Source: CAD feature listing. Evaluate the final solid. Frame: model axes, mm. Face numbers are marked on the shaded views. A direction names the side the tool comes from. Give positions to 0.01 mm unless a question says otherwise; leave off trailing zeros. Order: outer loops, then holes, each group sorted by start corner. A loop starts at its lowest first (then second) coordinate and runs counter-clockwise, first axis right, second up. Notation, with made-up numbers: M 87,34 L 129,34 A15 ccw 129,47 Z; hole C 64.25,20.5 d8. An arc over 180 degrees is marked long. Use CSV: the item, a comma, the result in double quotes. Start each with the question number.
Item 1: Pull-direction query (X, two-part tool) for the marked faces 1, 2, 3 and 4; classes: +X half, -X half, draft (parallel to the pull), parting line (faces both ways), or undercut.
Item 2: Section query C-C on x = 15. Count the separate pieces of the cut face and the enclosed holes in it, and give its area (3 significant figures).
Item 3: Access query for the marked faces 5, 6 and 7. Directions: +Z, -Z, +X, -X, +Y, -Y. A direction counts if a zero-diameter tool reaches every point of the face in a straight line with its end or side. Return the directions, or none.
Item 4: Section query B-B on y = -11.5. Return loops of the section in (x, z).
Item 5: Ray query, probe 1 along X at (y, z) = (-11.5, 1.3); probe 2 along Y at (x, z) = (0, 2.3); probe 3 along Y at (x, z) = (1, 2). Return the intervals inside material, ascending. Write a range as from..to.
Item 6: Section query A-A on x = -15.5. Return loops of the section in (y, z), and give its area (3 significant figures).
Item 7: First-contact query: pin 1 (4 mm diameter, centred on x = 10.5, y = -21.5, fed in from -Z); pin 2 (4.5 mm diameter, centred on x = 15.5, y = 19.5, fed in from +Z); pin 3 (4 mm diameter, centred on x = -15.5, y = -11.5, fed in from -Z); pin 4 (3 mm diameter, centred on x = 15.5, y = -11.5, fed in from -Z). Flat tips, straight axial feed; report the tip coordinate or a pass-through.
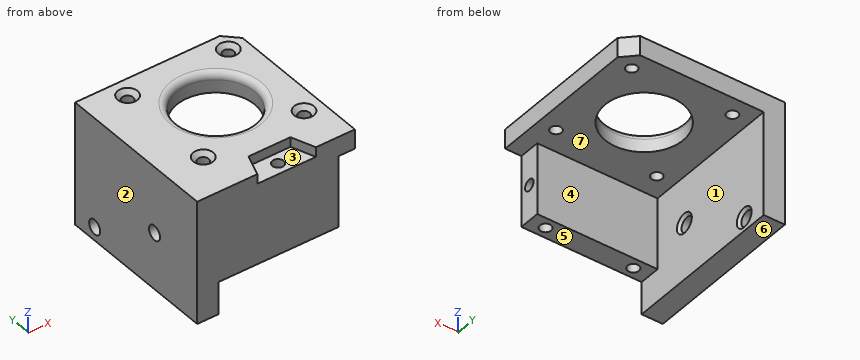
from build123d import *

# Parameters (mm, degrees)
SKETCH028_W         = 6.5
SKETCH028_H         = 50
PAD010_DEPTH        = 6
PAD010_DEPTH_BACK   = 32
HOLE011_D           = 4.5
HOLE011_DEPTH       = 25
HOLE011_CSINK_D     = 6.1
HOLE011_CSINK_ANGLE = 90
SKETCH_W            = 37
SKETCH_H            = 6.5
PAD_DEPTH           = 22
SKETCH041_R         = 1.75
POCKET_DEPTH        = 4
SKETCH042_R         = 1.75
POCKET014_DEPTH     = 3
BINDER016_W         = 50
BINDER016_H         = 42
PAD009_DEPTH        = 6
HOLE007_D           = 3.4
HOLE007_CSINK_D     = 6.1
HOLE007_CSINK_ANGLE = 90
SKETCH030_R         = 12
POCKET008_DEPTH     = 6.001
FILLET003_R         = 2
POCKET012_DEPTH     = 3
SKETCH040_R         = 1.75
POCKET013_DEPTH     = 3.001
CHAMFER_SIZE        = 4


with BuildPart() as obj1:
    # Sketch028 (on Face1 of Binder017) → Pad010 (new body, two sides)
    with BuildSketch(Plane.XY) as pad010_sk:
        with Locations((-24.25, 0)):
            Rectangle(SKETCH028_W, SKETCH028_H)
    extrude(amount=PAD010_DEPTH)
    extrude(pad010_sk.sketch, amount=-PAD010_DEPTH_BACK)

    # Hole011
    with Locations(Plane(origin=(-21, 25, -2), x_dir=(0, 1, 0), z_dir=(1, 0, 0))):
        with Locations((-32.5, -12.5), (-8, -25.81125)):
            CounterSinkHole(HOLE011_D / 2, HOLE011_CSINK_D / 2, depth=HOLE011_DEPTH, counter_sink_angle=HOLE011_CSINK_ANGLE)


with BuildPart() as obj2:
    # Sketch (on Face1 of Binder) → Pad (new body)
    with BuildSketch(Plane.XY):
        with Locations((-2.5, -21.75)):
            Rectangle(SKETCH_W, SKETCH_H)
    extrude(amount=-PAD_DEPTH)

    # Sketch041 (on Face6 of Pad) → Pocket (cut)
    with BuildSketch(Plane(origin=(0, 0, -22), x_dir=(1, 0, 0), z_dir=(0, 0, -1))):
        with Locations((-16, 21.75)):
            Circle(SKETCH041_R)
        with Locations((11, 21.75)):
            Circle(SKETCH041_R)
    extrude(amount=-POCKET_DEPTH, mode=Mode.SUBTRACT)

    # Sketch042 (on Face6 of Pocket) → Pocket014 (cut)
    with BuildSketch(Plane.YZ.offset(16)):
        with Locations((-21.75, -11)):
            Circle(SKETCH042_R)
    extrude(amount=-POCKET014_DEPTH, mode=Mode.SUBTRACT)


with BuildPart() as obj3:
    # Binder016 → Pad009 (new body)
    with BuildSketch(Plane(origin=(0, 0, 0), x_dir=(0, 1, 0), z_dir=(0, 0, 1))):
        Rectangle(BINDER016_W, BINDER016_H)
    extrude(amount=PAD009_DEPTH)

    # Hole007 (through all)
    with Locations(Plane.XY.offset(6)):
        with Locations((-15.5, 19.5), (-15.5, -11.5), (15.5, -11.5), (15.5, 19.5)):
            CounterSinkHole(HOLE007_D / 2, HOLE007_CSINK_D / 2, counter_sink_angle=HOLE007_CSINK_ANGLE)

    # Sketch030 (on Face5 of Hole007) → Pocket008 (cut, through all)
    with BuildSketch(Plane.XY.offset(6)):
        with Locations((0, 4)):
            Circle(SKETCH030_R)
    extrude(amount=-POCKET008_DEPTH, mode=Mode.SUBTRACT)

    # Fillet003
    fillet003_edges = [obj3.edges().sort_by_distance(p)[0] for p in [
        (-12, 4, 6),
    ]]
    fillet(fillet003_edges, radius=FILLET003_R)

    # Sketch031 (on Face1 of Fillet003) → Pocket012 (cut)
    with BuildSketch(Plane.XY.offset(6)):
        Polygon((-9, -25), (-6.452208, -18), (6.452208, -18), (9, -25), align=None)
    extrude(amount=-POCKET012_DEPTH, mode=Mode.SUBTRACT)

    # Sketch040 (on Face15 of Pocket012) → Pocket013 (cut, through all)
    with BuildSketch(Plane.XY.offset(3)):
        with Locations((0, -21.5)):
            Circle(SKETCH040_R)
    extrude(amount=-POCKET013_DEPTH, mode=Mode.SUBTRACT)

    # Chamfer
    chamfer_edges = [obj3.edges().sort_by_distance(p)[0] for p in [
        (21, 25, 3),
    ]]
    chamfer(chamfer_edges, length=CHAMFER_SIZE)

    # Fusion: union obj1, obj2
    add(obj1.part)
    add(obj2.part)


solid = obj3.part
Verdict:
1,face 1,"+X half"
1,face 2,"-X half"
1,face 3,"undercut"
1,face 4,"draft"
2,separate pieces,"3"
2,enclosed holes,"1"
2,area,"391 mm2"
3,face 5,"-Z, +X, +Y, -Y"
3,face 6,"-Z, +X, -X, +Y, -Y"
3,face 7,"-Z, +X, +Y"
4,outline,"M -27.5,-32 L -21,-32 L -21,0 L -17.2,0 L -17.2,4.65 L -18.55,6 L -27.5,6 Z; M -13.8,0 L 13.8,0 L 13.8,4.65 L 12.45,6 L -12.45,6 L -13.8,4.65 Z; M 17.2,0 L 21,0 L 21,6 L 18.55,6 L 17.2,4.65 Z"
5,probe 1,"-27.5..-17.2, -13.8..13.8, 17.2..21"
5,probe 2,"-25..-23.25, -19.75..-8, 16..25"
5,probe 3,"-25..-22.94, -20.06..-7.96, 15.96..25"
6,outline,"M -25,-22 L -23.43,-22 L -23.43,-18 L -20.07,-18 L -20.07,-22 L -18.5,-22 L -18.5,0 L -13.2,0 L -13.2,4.65 L -14.55,6 L -25,6 Z; M -9.8,0 L 17.8,0 L 17.8,4.65 L 16.45,6 L -8.45,6 L -9.8,4.65 Z; M 21.2,0 L 25,0 L 25,6 L 22.55,6 L 21.2,4.65 Z"
6,area,"385 mm2"
7,pin 1,"z = -22"
7,pin 2,"z = 5.2"
7,pin 3,"z = 0"
7,pin 4,"through"
